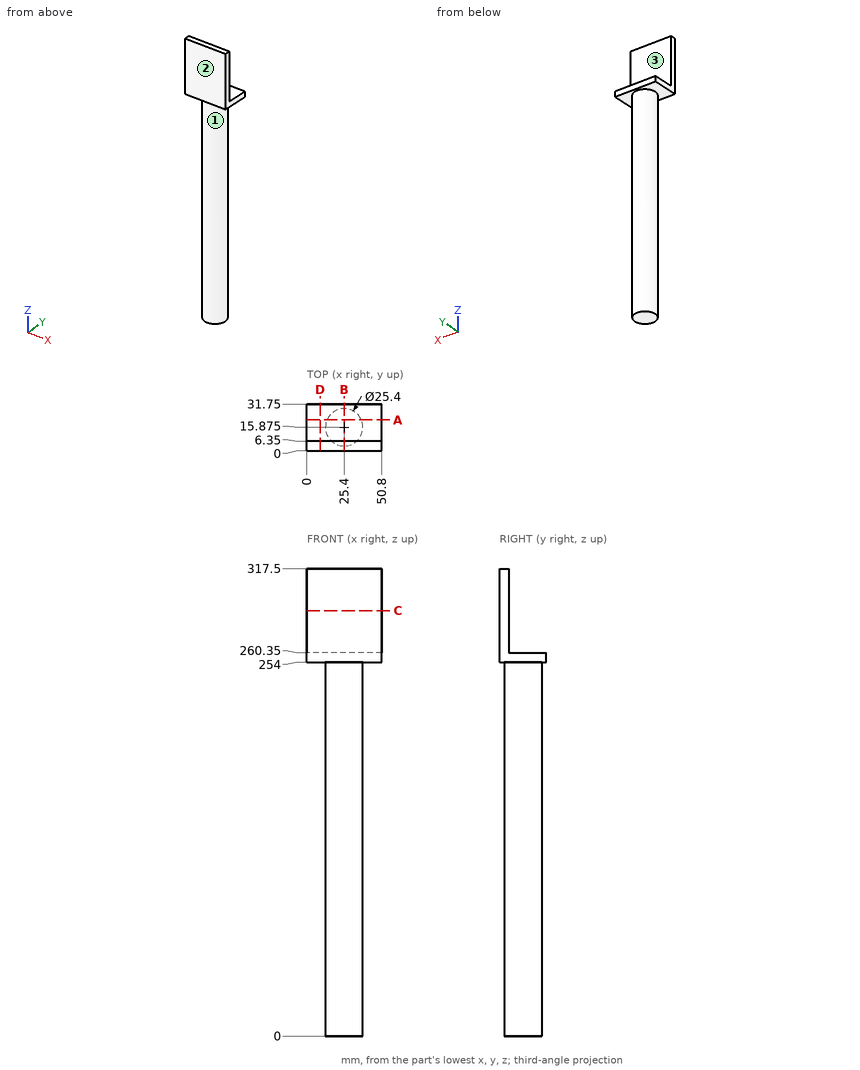
Answer from the drawing. Dimensions are ordinates in mm from the lowest x, y and z of the part. A direction names the side the tool comes from. Round coordinates to 2 decimals unless told otherwise and drop trailing zeros. Order: outer loops, then holes, each group sorted by start corner. A loop starts at its lowest first (then second) coordinate and runs counter-clockwise, first axis right, second up. Notation, with made-up numbers: (33, 29.5) -> (48, 29.5) arc R35 ccw to (48, 68.5) -> close; hole circle Ø4 at (33, 52.25). An arc over 180 degrees is marked (long way). Answer as CSV lines item,"result".
Q1. Which of the six approach directions +Z, -Z, +X, -X, +Y, -Y give full straight-line access (tool end or side, diameter ignored) to the marked faces 1, 2 and 3?
Computed values:
face 1,"-Z"
face 2,"+Z, -Z, +X, -X, -Y"
face 3,"+Z, +X, -X, +Y"
Q2. A cutting plane is placed at C-C on z = 289. Determine the outline of the cut face in (x, y), plus the area to 3 significant figures.
Computed values:
outline,"(0, 0) -> (50.8, 0) -> (50.8, 6.35) -> (0, 6.35) -> close"
area,"323 mm^2"
Q3. A cutting plane is placed at B-B on x = 25.4. Determine the outline of the cut face in (y, z) (3 decimals), plus the area to 3 significant figures.
Computed values:
outline,"(0, 254) -> (3.175, 254) -> (3.175, 0) -> (28.575, 0) -> (28.575, 254) -> (31.75, 254) -> (31.75, 260.35) -> (6.35, 260.35) -> (6.35, 317.5) -> (0, 317.5) -> close"
area,"7,020 mm^2"
Q4. Consider line 1 (Z direction, x = 36.5, y = 20.5); line 2 (Z direction, x = 3.5, y = 22); line 3 (X direction, y = 17, z = 166). Determine where each line is inside the solid, lowest interval first. Write a range as from..to.
Computed values:
line 1,"z = 0..260.35"
line 2,"z = 254..260.35"
line 3,"x = 12.75..38.05"
Q5. Given pin 1 (8 mm diameter, centred on x = 10, z = 150, fed in from +Y); pin 2 (8 mm diameter, centred on x = 38, z = 64.5, fed in from -Y); pin 3 (6 mm diameter, centred on x = 13, z = 124, fed in from +Y); pin 4 (9.5 mm diameter, centred on x = 29, y = 18, fed in from -Z), each flat-ended and moving along its own axis, determine where each tip first touches the part or whether it passes through.
Computed values:
pin 1,"stops at y = 21.47"
pin 2,"stops at y = 6.53"
pin 3,"stops at y = 24.41"
pin 4,"stops at z = 0"
Q6. A cutting plane is placed at D-D on x = 9. Determine the outline of the cut face in (y, z).
Computed values:
outline,"(0, 254) -> (31.75, 254) -> (31.75, 260.35) -> (6.35, 260.35) -> (6.35, 317.5) -> (0, 317.5) -> close"
Q7. A cutting plane is placed at A-A on y = 21. Determine the outline of the cut face in (x, z).
Computed values:
outline,"(0, 254) -> (13.78, 254) -> (13.78, 0) -> (37.02, 0) -> (37.02, 254) -> (50.8, 254) -> (50.8, 260.35) -> (0, 260.35) -> close"
